```python
from build123d import *

# Parameters (mm, degrees)
BOSS_EXTRUDE2_START = -50
BOSS_EXTRUDE2_DEPTH = 100
FILLET2_R           = 1
SKETCH11_OUTSIDE_W  = 76.321
SKETCH11_OUTSIDE_H  = 126.318
CUT_EXTRUDE6_DEPTH  = 50
SKETCH21_W          = 25.00380553
SKETCH21_H          = 54.5
CUT_EXTRUDE18_DEPTH = 50
SKETCH14_R          = 1.5
CUT_EXTRUDE14_DEPTH = 30
SKETCH15_R          = 4.15
CUT_EXTRUDE15_DEPTH = 30
SHELL2_START        = -31.45
SHELL2_DEPTH        = 62.9
SHELL2_START_2      = -17.78576348
SHELL2_2_DEPTH      = 43.889459003
SKETCH22_W          = 62.9
SKETCH22_H          = 17.053565945
SKETCH22_H_2        = 1.226371558
SKETCH22_H_3        = 0.669933019
CUT_EXTRUDE19_DEPTH = 23
SKETCH18_R          = 1.5
CUT_EXTRUDE16_DEPTH = 30
SKETCH19_R          = 1.5
CUT_EXTRUDE17_DEPTH = 15
BOSS_EXTRUDE3_DEPTH = 4


with BuildPart() as part:
    # Boss-Extrude2: read off the stored shape, not the designer's step
    # Boss-Extrude2 outline → Boss-Extrude2 (new body)
    with BuildSketch(Plane.XY.offset(BOSS_EXTRUDE2_START)):
        with BuildLine():
            Line((7.173376116, 28), (-17.826623884, 28))
            add(Edge.make_bspline(
                [(-17.826623884, 28), (-27.185874908, 27.50099933), (-35.223916981, 24.964377467), (-41.44802417, 19.674318155), (-45.338717867, 12.08134087), (-46.286792493, 3.622346125), (-43.873364855, -4.224078001), (-38.072691487, -10.630357441), (-29.305703518, -15.557723074), (-17.826623884, -19.78576348)],
                knots=[0, 0, 0, 0, 0, 0, 0, 0, 0, 0, 1, 1, 1, 1, 1, 1, 1, 1, 1, 1], degree=9))
            Line((-17.826623884, -19.78576348), (7.173376116, -19.78576348))
            Line((7.173376116, -19.78576348), (7.173376116, 28))
        make_face()
    extrude(amount=BOSS_EXTRUDE2_DEPTH)

    # Fillet2
    # the kernel refuses this fillet: 1 mm, written as the material it takes off along each edge
    with BuildSketch(Plane(origin=(9.673376116, 28, 50), x_dir=(0, 0, -1), z_dir=(-1, 0, 0))) as fillet2_piece_1:
        with BuildLine():
            CenterArc((FILLET2_R, FILLET2_R), FILLET2_R, 180, 90)
            Line((0, FILLET2_R), (0, 0))
            Line((0, 0), (FILLET2_R, 0))
        make_face()
    extrude(amount=35, mode=Mode.SUBTRACT)
    with BuildSketch(Plane(origin=(7.173376116, -22.28576348, 50), x_dir=(0, 0, -1), z_dir=(0, 1, 0))) as fillet2_piece_2:
        with BuildLine():
            CenterArc((FILLET2_R, FILLET2_R), FILLET2_R, 180, 90)
            Line((0, FILLET2_R), (0, 0))
            Line((0, 0), (FILLET2_R, 0))
        make_face()
    extrude(amount=52.78576348, mode=Mode.SUBTRACT)

    # Sketch11 outside → Cut-Extrude6 (cut, symmetric)
    with BuildSketch(Plane(origin=(0, 0, 0), x_dir=(1, 0, 0), z_dir=(0, 1, 0))):
        with Locations((-17.8285, 0)):
            Rectangle(SKETCH11_OUTSIDE_W, SKETCH11_OUTSIDE_H)
        Polygon((7.173376116, -33.45), (7.173376116, 33.45), (-17.826623884, 33.45), (-17.830429414, 29.25), (-42.830429414, 29.25), (-42.830429414, -29.25), (-17.830429414, -29.25), (-17.826623884, -33.45), align=None, mode=Mode.SUBTRACT)
    extrude(amount=CUT_EXTRUDE6_DEPTH, both=True, mode=Mode.SUBTRACT)

    # Sketch21 → Cut-Extrude18 (cut)
    with BuildSketch(Plane(origin=(0, 28, 0), x_dir=(1, 0, 0), z_dir=(0, 1, 0))):
        with Locations((-30.328526649, 0)):
            Rectangle(SKETCH21_W, SKETCH21_H)
    extrude(amount=-CUT_EXTRUDE18_DEPTH, mode=Mode.SUBTRACT)

    # Sketch14 → Cut-Extrude14 (cut)
    with BuildSketch(Plane.XY.offset(29.25)):
        with Locations((-30.330429414, -1.001364342)):
            Circle(SKETCH14_R)
        with Locations((-30.330429414, 5.998635658)):
            Circle(SKETCH14_R)
        with Locations((-37.330429414, 5.998635658)):
            Circle(SKETCH14_R)
        with Locations((-30.330429414, 12.998635658)):
            Circle(SKETCH14_R)
        with Locations((-23.330429414, 5.998635658)):
            Circle(SKETCH14_R)
    extrude(amount=-CUT_EXTRUDE14_DEPTH, mode=Mode.SUBTRACT)

    # Sketch15 → Cut-Extrude15 (cut)
    with BuildSketch(Plane(origin=(0, 0, -29.25), x_dir=(-1, 0, 0), z_dir=(0, 0, -1))):
        with Locations((30.330429414, 5.998635658)):
            Circle(SKETCH15_R)
    extrude(amount=-CUT_EXTRUDE15_DEPTH, mode=Mode.SUBTRACT)

    # Shell2: read off the stored shape, not the designer's step
    # Shell2 outline → Shell2 (cut)
    with BuildSketch(Plane.XY.offset(SHELL2_START)):
        with BuildLine():
            Line((7.173376116, -17.78576348), (7.173376116, 27.330066981))
            add(Edge.make_bspline(
                [(7.173376116, 27.330066981), (5.64775073, 27.248726274), (4.122125344, 27.167385568), (2.596499959, 27.086044862), (1.070874573, 27.004704155), (-0.454750813, 26.923363449), (-1.980376199, 26.842022743), (-3.506001584, 26.760682036), (-5.03162697, 26.67934133), (-6.557252356, 26.598000624), (-8.082877742, 26.516659917), (-9.608503127, 26.435319211), (-11.455719773, 26.336832447), (-11.777311032, 26.31968639), (-12.098902291, 26.302540333), (-12.420493551, 26.285394276), (-12.74208481, 26.268248218), (-13.06367607, 26.251102161), (-13.385267329, 26.233956104), (-13.706858589, 26.216810047), (-14.028449848, 26.199663989), (-14.350041108, 26.182517932), (-14.671632367, 26.165371875), (-15.062673648, 26.144522999), (-15.132123669, 26.140820181), (-15.201573691, 26.137117362), (-15.271023712, 26.133414544), (-15.340473734, 26.129711725), (-15.409923755, 26.126008907), (-15.479373777, 26.122306089), (-15.548823798, 26.11860327), (-15.61827382, 26.114900452), (-15.687723841, 26.111197633), (-15.757173863, 26.107494815), (-15.826623884, 26.103791996)],
                knots=[-0.295530754, -0.295530754, -0.295530754, -0.295530754, -0.295530754, -0.295530754, -0.295530754, -0.295530754, -0.295530754, -0.295530754, -0.295530754, -0.295530754, -0.295530754, -0.078187809, -0.078187809, -0.078187809, -0.078187809, -0.078187809, -0.078187809, -0.078187809, -0.078187809, -0.078187809, -0.078187809, -0.078187809, -0.032373422, -0.032373422, -0.032373422, -0.032373422, -0.032373422, -0.032373422, -0.032373422, -0.032373422, -0.032373422, -0.032373422, -0.032373422, -0.022479465, -0.022479465, -0.022479465, -0.022479465, -0.022479465, -0.022479465, -0.022479465, -0.022479465, -0.022479465, -0.022479465, -0.022479465, -0.022479465, -0.022479465], degree=12))
            Line((-15.826623884, 26.103791996), (-15.826623884, -17.78576348))
            Line((-15.826623884, -17.78576348), (7.173376116, -17.78576348))
        make_face()
    extrude(amount=SHELL2_DEPTH, mode=Mode.SUBTRACT)

    # Shell2 2 outline → Shell2 2 (cut)
    with BuildSketch(Plane(origin=(0, 0, 0), x_dir=(1, 0, 0), z_dir=(0, 1, 0)).offset(SHELL2_START_2)):
        Polygon((-15.830428593, 29.25), (-15.826623884, 29.25), (-15.826623884, 31.45), (-15.82843522, 31.45), align=None)
        Polygon((-15.826623884, -29.25), (-15.830428593, -29.25), (-15.82843522, -31.45), (-15.826623884, -31.45), align=None)
    extrude(amount=SHELL2_2_DEPTH, mode=Mode.SUBTRACT)

    # Sketch22 → Cut-Extrude19 (cut)
    with BuildSketch(Plane(origin=(7.173376116, 0, 0), x_dir=(0, 0, -1), z_dir=(1, 0, 0))):
        with Locations((0, 36.526782973)):
            Rectangle(SKETCH22_W, SKETCH22_H)
        with Locations((0, 26.716881202)):
            Rectangle(SKETCH22_W, SKETCH22_H_2)
        with Locations((0, 27.665033491)):
            Rectangle(SKETCH22_W, SKETCH22_H_3)
    extrude(amount=-CUT_EXTRUDE19_DEPTH, mode=Mode.SUBTRACT)

    # Sketch18 → Cut-Extrude16 (cut)
    with BuildSketch(Plane.ZY.offset(27.826623884)):
        with Locations(Location((0, 5.207061298, 0), (0, 0, 180))):
            Circle(SKETCH18_R)
        with Locations(Location((-9, 5.207061298, 0), (0, 0, 180))):
            Circle(SKETCH18_R)
        with Locations(Location((0, -3.792938702, 0), (0, 0, 180))):
            Circle(SKETCH18_R)
        with Locations(Location((9, 5.207061298, 0), (0, 0, 180))):
            Circle(SKETCH18_R)
        with Locations(Location((0, 14.207061298, 0), (0, 0, 180))):
            Circle(SKETCH18_R)
    extrude(amount=-CUT_EXTRUDE16_DEPTH, mode=Mode.SUBTRACT)

    # Sketch19 → Cut-Extrude17 (cut, symmetric)
    with BuildSketch(Plane(origin=(0, -17.78576348, 0), x_dir=(1, 0, 0), z_dir=(0, 1, 0))):
        with Locations(Location((4.274529249, -9.034575671, 0), (0, 0, 270))):
            Circle(SKETCH19_R)
        with Locations(Location((-2.725470751, -16.034575671, 0), (0, 0, 270))):
            Circle(SKETCH19_R)
        with Locations(Location((-9.725470751, -9.034575671, 0), (0, 0, 270))):
            Circle(SKETCH19_R)
        with Locations(Location((-2.725470751, -9.034575671, 0), (0, 0, 270))):
            Circle(SKETCH19_R)
        with Locations(Location((-2.725470751, 16.134575671, 0), (0, 0, 270))):
            Circle(SKETCH19_R)
        with Locations(Location((4.274529249, 9.134575671, 0), (0, 0, 270))):
            Circle(SKETCH19_R)
        with Locations(Location((-2.725470751, 2.134575671, 0), (0, 0, 270))):
            Circle(SKETCH19_R)
        with Locations(Location((-9.725470751, 9.134575671, 0), (0, 0, 270))):
            Circle(SKETCH19_R)
        with Locations(Location((-2.725470751, 9.134575671, 0), (0, 0, 270))):
            Circle(SKETCH19_R)
        with Locations(Location((-2.725470751, -2.034575671, 0), (0, 0, 270))):
            Circle(SKETCH19_R)
    extrude(amount=CUT_EXTRUDE17_DEPTH, both=True, mode=Mode.SUBTRACT)

    # Sketch20 → Boss-Extrude3 (add)
    with BuildSketch(Plane(origin=(7.173376116, 0, 0), x_dir=(0, 0, -1), z_dir=(1, 0, 0))):
        Polygon((-31.45, -17.78576348), (-31.45, 28), (-33.45, 28), (-33.45, -19.78576348), (33.45, -19.78576348), (33.45, 28), (31.45, 28), (31.45, -17.78576348), align=None)
    extrude(amount=BOSS_EXTRUDE3_DEPTH)


solid = part.part
```
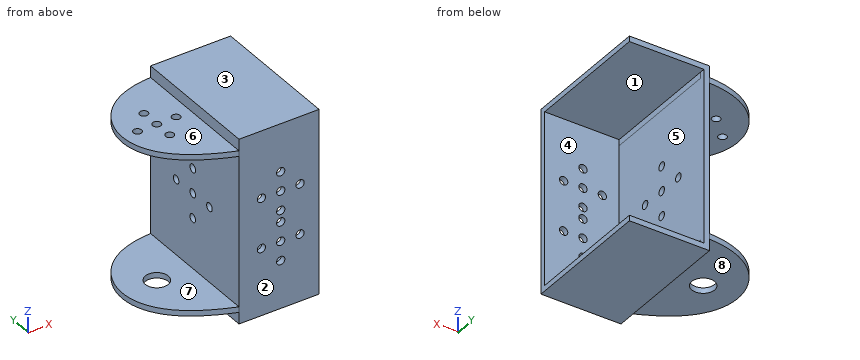
Input: part model. Units: mm. Frame: model coordinates. Face numbers are marked on the shaded views. A direction names the side the tool comes from. Give positions to 0.01 mm unless a question says otherwise; leave off trailing zeros. Loops run counter-clockwise (first coordinate to the right, second up) from the corner with the lowest first, then second, coordinate; pieces in that order, holes last. Notation, with made-up numbers: (35, 80) -> (69, 80) arc R19 ccw to (69, 88) -> close; hole circle Ø6 at (4, 8.5). An arc over 180 degrees is marked (long way). Use a Markdown table: item, result.
Q1. Section query B-B, the plane z = 5.5. Return the cut outline in (x, y).
Entries:
| item | result |
|---|---|
| outline | (-17.83, -19.79) -> (11.17, -19.79) -> (11.17, -17.79) -> (-15.83, -17.79) -> (-15.83, 28) -> (-17.83, 28) -> close |
Q2. Ray query, probe 1 along Y at (x, z) = (-16.55, 0); probe 2 along Z at (x, y) = (-39.5, 15); probe 3 along Z at (x, y) = (4.5, 25). Return the intervals inside material, ascending. Write a range as from..to.
Entries:
| item | result |
|---|---|
| probe 1 | y = -19.79..-5.29, -2.29..3.71, 6.71..12.71, 15.71..28 |
| probe 2 | z = -29.25..-27.25, 27.25..29.25 |
| probe 3 | z = -33.45..-31.45, 31.45..33.45 |
Q3. Section query C-C, the plane x = -37. State how many separate pieces and enclosed holes the cut face has, plus the area to 3 significant figures.
Entries:
| item | result |
|---|---|
| separate pieces | 3 |
| enclosed holes | 0 |
| area | 108 mm² |
Q4. Pull-direction query (Z, two-part tool) for the marked faces 1, 2, 3 and 4; classes: pulls with the +Z half, pulls with the -Z half, needs draft (parallel to the pull), parting line crosses it, or undercut.
Entries:
| item | result |
|---|---|
| face 1 | undercut |
| face 2 | needs draft |
| face 3 | pulls with the +Z half |
| face 4 | undercut |
Q5. Access query for the marked faces 5, 6, 7 and 8. Directions: +Z, -Z, +X, -X, +Y, -Y. A direction counts if a zero-diameter tool reaches every point of the face in a straight line with its end or side. Return the directions, or none.
Entries:
| item | result |
|---|---|
| face 5 | +X, +Y |
| face 6 | +Z, -X, +Y, -Y |
| face 7 | -X, +Y, -Y |
| face 8 | -Z, -X, +Y, -Y |
Q6. First-contact query: P1, Ø10, axis at y = -10, z = -4.5, coming from the -X side; P2, Ø12.5, axis at x = -33.5, y = 4, coming from the -Z side; P3, Ø21.5, axis at x = -4.5, z = -4.5, coming from the +Y side; P4, Ø3.5, axis at x = -2.73, z = 2.03, coming from the -Y side. Flat tips, straight axial feed; report the tip coordinate or a pass-through.
Entries:
| item | result |
|---|---|
| P1 | stops at x = -17.83 |
| P2 | stops at z = -29.25 |
| P3 | stops at y = -17.79 |
| P4 | stops at y = -19.79 |
Q7. Section query A-A, the plane z = -9. Return the cut outline in (x, y).
Entries:
| item | result |
|---|---|
| outline | (-17.83, -19.79) -> (-11.22, -19.79) -> (-11.22, -17.79) -> (-15.83, -17.79) -> (-15.83, 3.71) -> (-17.83, 3.71) -> close; (-17.83, 6.71) -> (-15.83, 6.71) -> (-15.83, 28) -> (-17.83, 28) -> close; (-8.23, -19.79) -> (-4.22, -19.79) -> (-4.22, -17.79) -> (-8.23, -17.79) -> close; (-1.23, -19.79) -> (2.78, -19.79) -> (2.78, -17.79) -> (-1.23, -17.79) -> close; (5.77, -19.79) -> (11.17, -19.79) -> (11.17, -17.79) -> (5.77, -17.79) -> close |
